from build123d import *

# Parameters (mm, degrees)
SKETCH1_W           = 154
SKETCH1_H           = 91.2
BOSS_EXTRUDE1_DEPTH = 2.9
CUT_EXTRUDE3_DEPTH  = 1.5


with BuildPart() as part:
    # Sketch1 → Boss-Extrude1 (new body)
    with BuildSketch(Plane.XY):
        with BuildLine():
            Line((99.87625, 76.6), (-94.12375, 76.6))
            ThreePointArc((-94.12375, 76.6), (-101.901924593, 73.378174593), (-105.12375, 65.6))
            Line((-105.12375, 65.6), (-105.12375, -65.6))
            ThreePointArc((-105.12375, -65.6), (-101.901924593, -73.378174593), (-94.12375, -76.6))
            Line((-94.12375, -76.6), (99.87625, -76.6))
            ThreePointArc((99.87625, -76.6), (107.654424593, -73.378174593), (110.87625, -65.6))
            Line((110.87625, -65.6), (110.87625, 65.6))
            ThreePointArc((110.87625, 65.6), (107.654424593, 73.378174593), (99.87625, 76.6))
        make_face()
        with Locations((2.87625, 0)):
            Rectangle(SKETCH1_W, SKETCH1_H, mode=Mode.SUBTRACT)
    extrude(amount=BOSS_EXTRUDE1_DEPTH)

    # Sketch2 → Cut-Extrude3 (cut)
    with BuildSketch(Plane.XY):
        with BuildLine():
            Line((99.87625, 75.6), (-94.12375, 75.6))
            ThreePointArc((-94.12375, 75.6), (-101.194817812, 72.671067812), (-104.12375, 65.6))
            Line((-104.12375, 65.6), (-104.12375, -65.6))
            ThreePointArc((-104.12375, -65.6), (-101.194817812, -72.671067812), (-94.12375, -75.6))
            Line((-94.12375, -75.6), (99.87625, -75.6))
            ThreePointArc((99.87625, -75.6), (106.947317812, -72.671067812), (109.87625, -65.6))
            Line((109.87625, -65.6), (109.87625, 65.6))
            ThreePointArc((109.87625, 65.6), (106.947317812, 72.671067812), (99.87625, 75.6))
        make_face()
        with BuildLine():
            Line((99.87625, 73.6), (-94.12375, 73.6))
            ThreePointArc((-94.12375, 73.6), (-99.780604249, 71.256854249), (-102.12375, 65.6))
            Line((-102.12375, 65.6), (-102.12375, -65.6))
            ThreePointArc((-102.12375, -65.6), (-99.780604249, -71.256854249), (-94.12375, -73.6))
            Line((-94.12375, -73.6), (99.87625, -73.6))
            ThreePointArc((99.87625, -73.6), (105.533104249, -71.256854249), (107.87625, -65.6))
            Line((107.87625, -65.6), (107.87625, 65.6))
            ThreePointArc((107.87625, 65.6), (105.533104249, 71.256854249), (99.87625, 73.6))
        make_face(mode=Mode.SUBTRACT)
    extrude(amount=CUT_EXTRUDE3_DEPTH, mode=Mode.SUBTRACT)


solid = part.part
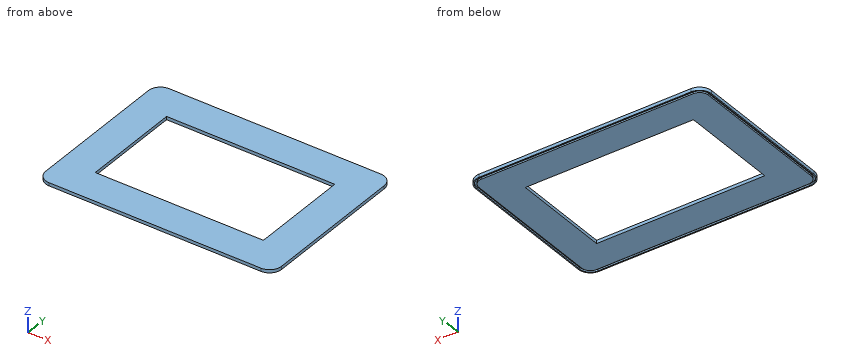
Can you work these out from the model? Positions are in its coordinate system, mm. Coordinates: 2 decimals unless noted, no trailing zeros. Loops run counter-clockwise (first coordinate to the right, second up) from the corner with the lowest first, then second, coordinate; pieces in that order, holes last. Notation, with made-up numbers: (7, 6) - (37, 6) arc R7 ccw to (37, 17) - close; hole circle Ø5 at (-11, 34). An arc over 180 degrees is marked (long way). Answer as a JSON object with one key per item and string values. Group by question number.
Item 1: If I drill on L1, parallel to X at y = 8.5, z = 1.25; L2, parallel to Y at x = -47.5, z = 1.4; L3, parallel to Y at x = -75, z = 0.8, over which ranges is the centre line in solid material (lowest first)? Write a range as from..to.
Item 2: If we section it at C-C (x = 46): List the corners of the cut face in (y, z) for me, plus the area to 3 significant figures.
Item 3: If we section it at B-B (z = 1.05): List the corners of the cut face in (x, y) for me, plus the area to 3 significant figures.
Item 4: If we section it at A-A (y = -32.5): List the corners of the cut face in (x, z) for me.
Returned:
{
 "1": {"L1": "x = -105.12..-104.12, -102.12..-74.12, 79.88..107.88, 109.88..110.88", "L2": "y = -76.6..-75.6, -73.6..-45.6, 45.6..73.6, 75.6..76.6", "L3": "y = -76.6..-75.6, -73.6..73.6, 75.6..76.6"},
 "2": {"outline": "(-76.6, 0) - (-75.6, 0) - (-75.6, 1.5) - (-73.6, 1.5) - (-73.6, 0) - (-45.6, 0) - (-45.6, 2.9) - (-76.6, 2.9) - close; (45.6, 0) - (73.6, 0) - (73.6, 1.5) - (75.6, 1.5) - (75.6, 0) - (76.6, 0) - (76.6, 2.9) - (45.6, 2.9) - close", "area": "174 mm²"},
 "3": {"outline": "(-105.12, -65.6) arc R11 ccw to (-94.12, -76.6) - (99.88, -76.6) arc R11 ccw to (110.88, -65.6) - (110.88, 65.6) arc R11 ccw to (99.88, 76.6) - (-94.12, 76.6) arc R11 ccw to (-105.12, 65.6) - close; (-102.12, -65.6) arc R8 ccw to (-94.12, -73.6) - (99.88, -73.6) arc R8 ccw to (107.88, -65.6) - (107.88, 65.6) arc R8 ccw to (99.88, 73.6) - (-94.12, 73.6) arc R8 ccw to (-102.12, 65.6) - close; hole (-104.12, -65.6) arc R10 ccw to (-94.12, -75.6) - (99.88, -75.6) arc R10 ccw to (109.88, -65.6) - (109.88, 65.6) arc R10 ccw to (99.88, 75.6) - (-94.12, 75.6) arc R10 ccw to (-104.12, 65.6) - close; hole (-74.12, -45.6) - (79.88, -45.6) - (79.88, 45.6) - (-74.12, 45.6) - close", "area": "17,500 mm²"},
 "4": {"outline": "(-105.12, 0) - (-104.12, 0) - (-104.12, 1.5) - (-102.12, 1.5) - (-102.12, 0) - (-74.12, 0) - (-74.12, 2.9) - (-105.12, 2.9) - close; (79.88, 0) - (107.88, 0) - (107.88, 1.5) - (109.88, 1.5) - (109.88, 0) - (110.88, 0) - (110.88, 2.9) - (79.88, 2.9) - close"}
}
